Here's how the part is built. I have some questions about the finished solid (model axes, mm). A direction names the side the tool comes from. Round coordinates to 2 decimals unless told otherwise and drop trailing zeros. Write each loop counter-clockwise with the first axis right and the second up, starting at its lowest first coordinate (ties: lowest second). Pieces come first, ordered by that corner, then holes. Notation, with made-up numbers: (-4, 48.25) -> (51, 48.25) arc R20 cw to (51, 83.25) -> close; hole circle Ø7 at (16, 72.25). An arc over 180 degrees is marked (long way). Put each result on its own line as item: value. Start each with the question number.
1. Suppose I cut it at B-B (x = 14.75). Please give me the cut outline in (y, z), then the cut area to 3 significant figures.
2. Suppose I cut it at D-D (x = 7). Please give me the cut outline in (y, z).
3. Suppose I cut it at C-C (y = 23). Please give me the cut outline in (x, z).
4. For pin 1 (8 mm diameter, centred on y = 25, z = 22, fed in from +X), with a flat end and sliding along its axis, tell me the tip position at first contact or that it passes through.
5. Which directions (+Z, -Z, +X, -X, +Y, -Y) give clear straight access to the entire face, cutting with the end or side of a thin tool? Please do faces 4 (the face through (2, 17, 15)), 5 (the face through (1.5, 16.1, 30)).
6. I need wall thicknesses on probe 1 along Y at (x, z) = (4.75, 12); probe 2 along X at (y, z) = (0.8, 15); probe 3 along Z at (x, y) = (7, 1.25). Which ranges of each line are inside material? Lowest first, please. Write a range as from..to.
7. We'd pull the mould along X, two halves only. Please class faces 1 (the face through (17, 1, 15)), 2 (the face through (9.31, 33.99, 14.04)), 3 (the face through (1.01, 24.69, 16.84)): +X half, -X half, draft (parallel to the pull), parting line (faces both ways), or undercut.
8. Suppose I cut it at A-A (z = 15). Please give me the cut outline in (x, y).
```python
from build123d import *

# Parameters (mm, degrees)
BOSS_EXTRUDE1_DEPTH = 30
SKETCH2_R           = 2.5
CUT_EXTRUDE1_DEPTH  = 10
SKETCH3_R           = 2.5
CUT_EXTRUDE2_DEPTH  = 10
SKETCH4_W           = 2
SKETCH4_H           = 30
BOSS_EXTRUDE2_DEPTH = 5
SKETCH5_W           = 17
SKETCH5_H           = 30
BOSS_EXTRUDE3_DEPTH = 2
SKETCH6_R           = 2.5
CUT_EXTRUDE3_DEPTH  = 2


with BuildPart() as part:
    # Sketch1 → Boss-Extrude1 (new body)
    with BuildSketch(Plane.XY):
        Polygon((0, 0), (0, 28), (2, 28), (2, 2), (17, 2), (17, 0), align=None)
    extrude(amount=BOSS_EXTRUDE1_DEPTH)

    # Sketch2 → Cut-Extrude1 (cut)
    with BuildSketch(Plane(origin=(0, 2, 0), x_dir=(1, 0, 0), z_dir=(0, 1, 0))):
        with Locations((7, -15)):
            Circle(SKETCH2_R)
    extrude(amount=-CUT_EXTRUDE1_DEPTH, mode=Mode.SUBTRACT)

    # Sketch3 → Cut-Extrude2 (cut)
    with BuildSketch(Plane(origin=(2, 0, 0), x_dir=(0, 0, -1), z_dir=(1, 0, 0))):
        with Locations((-15, 23)):
            Circle(SKETCH3_R)
    extrude(amount=-CUT_EXTRUDE2_DEPTH, mode=Mode.SUBTRACT)

    # Sketch4 → Boss-Extrude2 (add)
    with BuildSketch(Plane(origin=(0, 28, 0), x_dir=(1, 0, 0), z_dir=(0, 1, 0))):
        with Locations((1, -15)):
            Rectangle(SKETCH4_W, SKETCH4_H)
    extrude(amount=BOSS_EXTRUDE2_DEPTH)

    # Sketch5 → Boss-Extrude3 (add)
    with BuildSketch(Plane(origin=(0, 33, 0), x_dir=(1, 0, 0), z_dir=(0, 1, 0))):
        with Locations((8.5, -15)):
            Rectangle(SKETCH5_W, SKETCH5_H)
    extrude(amount=BOSS_EXTRUDE3_DEPTH)

    # Sketch6 → Cut-Extrude3 (cut)
    with BuildSketch(Plane.XZ.offset(-33)):
        with Locations((7, 15)):
            Circle(SKETCH6_R)
    extrude(amount=-CUT_EXTRUDE3_DEPTH, mode=Mode.SUBTRACT)


solid = part.part
```
Verdict:
1. outline: (0, 0) -> (2, 0) -> (2, 30) -> (0, 30) -> close; (33, 0) -> (35, 0) -> (35, 30) -> (33, 30) -> close
1. area: 120 mm^2
2. outline: (0, 0) -> (2, 0) -> (2, 12.5) -> (0, 12.5) -> close; (0, 17.5) -> (2, 17.5) -> (2, 30) -> (0, 30) -> close; (33, 0) -> (35, 0) -> (35, 12.5) -> (33, 12.5) -> close; (33, 17.5) -> (35, 17.5) -> (35, 30) -> (33, 30) -> close
3. outline: (0, 0) -> (2, 0) -> (2, 12.5) -> (0, 12.5) -> close; (0, 17.5) -> (2, 17.5) -> (2, 30) -> (0, 30) -> close
4. pin 1: stops at x = 2
5. face 4: +Z, -Z, +X
5. face 5: +Z, +X, -X, +Y, -Y
6. probe 1: y = 0..2, 33..35
6. probe 2: x = 0..4.5, 9.5..17
6. probe 3: z = 0..12.5, 17.5..30
7. face 1: +X half
7. face 2: undercut
7. face 3: draft
8. outline: (0, 0) -> (4.5, 0) -> (4.5, 2) -> (2, 2) -> (2, 20.5) -> (0, 20.5) -> close; (0, 25.5) -> (2, 25.5) -> (2, 33) -> (4.5, 33) -> (4.5, 35) -> (0, 35) -> close; (9.5, 0) -> (17, 0) -> (17, 2) -> (9.5, 2) -> close; (9.5, 33) -> (17, 33) -> (17, 35) -> (9.5, 35) -> close
